```python
from build123d import *

# Parameters (mm, degrees)
SKETCH1_W                            = 159.7
SKETCH1_H                            = 109.7
SKETCH1_W_2                          = 143.7
SKETCH1_H_2                          = 102.7
BOSS_EXTRUDE1_DEPTH                  = 6
F_2_4_2_4_DIAMETER_HOLE1_D           = 2.4
CUT_EXTRUDE10_DEPTH                  = 2.2
LPATTERN1_COUNT                      = 2
LPATTERN1_PITCH                      = 72
MIRROR2_COPY_1_DEPTH                 = 2.2
M2X0_4_TAPPED_HOLE1_D                = 1.6
M2X0_4_TAPPED_HOLE1_DEPTH            = 3.5
M2X0_4_TAPPED_HOLE1_CSINK_D          = 2.05
M2X0_4_TAPPED_HOLE1_CSINK_ANGLE      = 90
M2X0_4_TAPPED_HOLE1_TIP              = 0.480688495
CUT_EXTRUDE3_DEPTH                   = 0.5
SKETCH11_W                           = 4.35
SKETCH11_H                           = 6
CUT_EXTRUDE4_DEPTH                   = 2.2
CUT_EXTRUDE11_DEPTH                  = 97.948362544
CUT_EXTRUDE11_DEPTH_BACK             = 97.948362544
F_2_4_2_4_DIAMETER_HOLE2_D           = 2.4
F_2_7_2_7_DIAMETER_HOLE1_D           = 2.7
F_2_7_2_7_DIAMETER_HOLE1_CSINK_D     = 2.75
F_2_7_2_7_DIAMETER_HOLE1_CSINK_ANGLE = 90
CUT_EXTRUDE6_DEPTH                   = 98.059492065
SKETCH19_R                           = 1.4
CUT_EXTRUDE7_DEPTH                   = 3.5
SKETCH32_R                           = 1.375
BOSS_EXTRUDE2_DEPTH                  = 1
CUT_EXTRUDE8_DEPTH                   = 98.126438213
SKETCH8_R                            = 8
CUT_EXTRUDE9_DEPTH                   = 98.126438213
FILLET1_R                            = 2
FILLET2_R                            = 8
FILLET3_R                            = 1
FILLET4_R                            = 2
FILLET5_R                            = 0.5
SKETCH31_W                           = 48
SKETCH31_H                           = 1.6
CUT_EXTRUDE12_DEPTH                  = 98.126438213
CHAMFER1_START                       = -1
CHAMFER1_DEPTH                       = 8
CHAMFER1_2_DEPTH                     = 6
FILLET6_R                            = 2


with BuildPart() as part:
    # Sketch1 → Boss-Extrude1 (new body)
    with BuildSketch(Plane(origin=(0, 0, 0), x_dir=(1, 0, 0), z_dir=(0, 1, 0))):
        Rectangle(SKETCH1_W, SKETCH1_H)
        Rectangle(SKETCH1_W_2, SKETCH1_H_2, mode=Mode.SUBTRACT)
    extrude(amount=BOSS_EXTRUDE1_DEPTH)

    # Ø2.4 (2.4) Diameter Hole1 (through all)
    with Locations(Plane(origin=(0, 6, 0), x_dir=(1, 0, 0), z_dir=(0, 1, 0))):
        with Locations((-77.5, 36), (77.5, 36), (-77.5, -36), (77.5, -36)):
            Hole(F_2_4_2_4_DIAMETER_HOLE1_D / 2)

    # Sketch29 → Cut-Extrude10 (cut)
    with BuildSketch(Plane(origin=(0, 6, 0), x_dir=(1, 0, 0), z_dir=(0, 1, 0))):
        with BuildLine():
            Line((-77.5, 38), (-79.85, 38))
            Line((-79.85, 38), (-79.85, 34))
            Line((-79.85, 34), (-77.5, 34))
            ThreePointArc((-77.5, 34), (-75.5, 36), (-77.5, 38))
        make_face()
    cut_extrude10 = extrude(amount=-CUT_EXTRUDE10_DEPTH, mode=Mode.SUBTRACT)

    # LPattern1: Cut-Extrude10 ×2
    with Locations(*[(0, 0, i * LPATTERN1_PITCH) for i in range(1, LPATTERN1_COUNT)]):
        add(cut_extrude10, mode=Mode.SUBTRACT)

    # Mirror2: Cut-Extrude10 across plane
    add(cut_extrude10.mirror(Plane(origin=(0, 0, 0), x_dir=(0, 0, 1), z_dir=(1, 0, 0))), mode=Mode.SUBTRACT)

    # Mirror2 copy 1 sketch → Mirror2 copy 1 (cut)
    with BuildSketch(Plane(origin=(0, 6, 72), x_dir=(-1, 0, 0), z_dir=(0, 1, 0))):
        with BuildLine():
            Line((-77.5, -38), (-79.85, -38))
            Line((-79.85, -38), (-79.85, -34))
            Line((-79.85, -34), (-77.5, -34))
            ThreePointArc((-77.5, -34), (-75.5, -36), (-77.5, -38))
        make_face()
    extrude(amount=-MIRROR2_COPY_1_DEPTH, mode=Mode.SUBTRACT)

    # M2x0.4 Tapped Hole1
    with Locations(Plane(origin=(0, 6, 0), x_dir=(1, 0, 0), z_dir=(0, 1, 0))):
        with Locations((-74, 40), (-74, -40), (74, 40), (74, -40)):
            CounterSinkHole(M2X0_4_TAPPED_HOLE1_D / 2, M2X0_4_TAPPED_HOLE1_CSINK_D / 2, depth=M2X0_4_TAPPED_HOLE1_DEPTH, counter_sink_angle=M2X0_4_TAPPED_HOLE1_CSINK_ANGLE)
            with Locations((0, 0, -(M2X0_4_TAPPED_HOLE1_DEPTH + M2X0_4_TAPPED_HOLE1_TIP / 2))):  # 118° drill point
                Cone(0, M2X0_4_TAPPED_HOLE1_D / 2, M2X0_4_TAPPED_HOLE1_TIP, mode=Mode.SUBTRACT)

    # Sketch9 → Cut-Extrude3 (cut)
    with BuildSketch(Plane(origin=(0, 6, 0), x_dir=(1, 0, 0), z_dir=(0, 1, 0))):
        with BuildLine():
            Line((-74.85, 4), (-74.85, -4))
            ThreePointArc((-74.85, -4), (-76.85, -6), (-78.85, -4))
            Line((-78.85, -4), (-78.85, 4))
            ThreePointArc((-78.85, 4), (-76.85, 6), (-74.85, 4))
        make_face()
    cut_extrude3 = extrude(amount=-CUT_EXTRUDE3_DEPTH, mode=Mode.SUBTRACT)

    # Mirror1: Cut-Extrude3 across plane
    add(cut_extrude3.mirror(Plane(origin=(0, 0, 0), x_dir=(0, 0, 1), z_dir=(1, 0, 0))), mode=Mode.SUBTRACT)

    # Sketch11 → Cut-Extrude4 (cut)
    with BuildSketch(Plane(origin=(0, 6, 0), x_dir=(1, 0, 0), z_dir=(0, 1, 0))):
        with Locations((-77.675, 39)):
            Rectangle(SKETCH11_W, SKETCH11_H)
    extrude(amount=-CUT_EXTRUDE4_DEPTH, mode=Mode.SUBTRACT)

    # Sketch30 → Cut-Extrude11 (cut, two sides: drawn at the far end of the back side and taken through both)
    with BuildSketch(Plane(origin=(0, 3.8, 0), x_dir=(1, 0, 0), z_dir=(0, 1, 0)).offset(-CUT_EXTRUDE11_DEPTH_BACK)):
        with BuildLine():
            Line((-75.5, 40), (-75.5, 42))
            Line((-75.5, 42), (-79.85, 42))
            Line((-79.85, 42), (-79.85, 38))
            Line((-79.85, 38), (-77.5, 38))
            ThreePointArc((-77.5, 38), (-76.085786438, 38.585786438), (-75.5, 40))
        make_face()
    extrude(amount=CUT_EXTRUDE11_DEPTH + CUT_EXTRUDE11_DEPTH_BACK, mode=Mode.SUBTRACT)

    # Ø2.4 (2.4) Diameter Hole2 (through all)
    with Locations(Plane(origin=(0, 6, 0), x_dir=(1, 0, 0), z_dir=(0, 1, 0))):
        with Locations((-77.5, -40), (77.5, 40), (77.5, -40)):
            Hole(F_2_4_2_4_DIAMETER_HOLE2_D / 2)

    # Ø2.7 (2.7) Diameter Hole1 (through all)
    with Locations(Plane(origin=(0, 6, 0), x_dir=(1, 0, 0), z_dir=(0, 1, 0))):
        with Locations((-77.5, 29), (-77.5, -29), (77.5, 29), (77.5, -29)):
            CounterSinkHole(F_2_7_2_7_DIAMETER_HOLE1_D / 2, F_2_7_2_7_DIAMETER_HOLE1_CSINK_D / 2, counter_sink_angle=F_2_7_2_7_DIAMETER_HOLE1_CSINK_ANGLE)

    # Sketch18 → Cut-Extrude6 (cut, through all)
    with BuildSketch(Plane(origin=(0, 6, 0), x_dir=(1, 0, 0), z_dir=(0, 1, 0))):
        with BuildLine():
            Line((-78.85, 24.85), (-79.85, 24.85))
            Line((-79.85, 24.85), (-79.85, 18.85))
            Line((-79.85, 18.85), (-78.85, 18.85))
            ThreePointArc((-78.85, 18.85), (-77.435786438, 19.435786438), (-76.85, 20.85))
            Line((-76.85, 20.85), (-76.85, 22.85))
            ThreePointArc((-76.85, 22.85), (-77.435786438, 24.264213562), (-78.85, 24.85))
        make_face()
    extrude(amount=-CUT_EXTRUDE6_DEPTH, mode=Mode.SUBTRACT)

    # Sketch19 → Cut-Extrude7 (cut)
    with BuildSketch(Plane(origin=(0, 6, 0), x_dir=(1, 0, 0), z_dir=(0, 1, 0))):
        with Locations(Location((77.35, 44.85, 0), (0, 0, 270))):
            Circle(SKETCH19_R)
        with Locations(Location((-77.35, -44.85, 0), (0, 0, 270))):
            Circle(SKETCH19_R)
    extrude(amount=-CUT_EXTRUDE7_DEPTH, mode=Mode.SUBTRACT)

    # Sketch32 → Boss-Extrude2 (add)
    with BuildSketch(Plane.XZ):
        with Locations(Location((-77.35, 44.85, 0), (0, 0, 90))):
            Circle(SKETCH32_R)
        with Locations(Location((77.35, -44.85, 0), (0, 0, 90))):
            Circle(SKETCH32_R)
    extrude(amount=BOSS_EXTRUDE2_DEPTH)

    # Sketch7 → Cut-Extrude8 (cut, through all)
    with BuildSketch(Plane(origin=(0, 6, 0), x_dir=(1, 0, 0), z_dir=(0, 1, 0))):
        with BuildLine():
            Line((-76.85, 48.85), (-79.85, 48.85))
            Line((-79.85, 48.85), (-79.85, 40.85))
            Line((-79.85, 40.85), (-76.85, 40.85))
            ThreePointArc((-76.85, 40.85), (-72.85, 44.85), (-76.85, 48.85))
        make_face()
    extrude(amount=-CUT_EXTRUDE8_DEPTH, mode=Mode.SUBTRACT)

    # Sketch8 → Cut-Extrude9 (cut, through all)
    with BuildSketch(Plane(origin=(0, 6, 0), x_dir=(1, 0, 0), z_dir=(0, 1, 0))):
        with Locations((-79.85, -54.85)):
            Circle(SKETCH8_R)
    extrude(amount=-CUT_EXTRUDE9_DEPTH, mode=Mode.SUBTRACT)

    # Fillet1
    fillet1_edges = [part.edges().sort_by_distance(p)[0] for p in [
        (71.85, 3, 51.35),
        (71.85, 3, -51.35),
        (-71.85, 3, -51.35),
        (-71.85, 3, 51.35),
    ]]
    fillet(fillet1_edges, radius=FILLET1_R)

    # Fillet2
    # the kernel refuses this fillet: 8 mm, written as the material it takes off along each edge
    with BuildSketch(Plane(origin=(79.85, -20, 54.85), x_dir=(-1, 0, 0), z_dir=(0, 1, 0)), Plane(origin=(79.85, -20, -54.85), x_dir=(0, 0, 1), z_dir=(0, 1, 0))) as fillet2_piece_1:
        with BuildLine():
            CenterArc((FILLET2_R, -FILLET2_R), FILLET2_R, 90, 90)
            Line((0, -FILLET2_R), (-FILLET2_R * 0.02, -FILLET2_R))
            Line((-FILLET2_R * 0.02, -FILLET2_R), (-FILLET2_R * 0.02, FILLET2_R * 0.02))
            Line((-FILLET2_R * 0.02, FILLET2_R * 0.02), (FILLET2_R, FILLET2_R * 0.02))
            Line((FILLET2_R, FILLET2_R * 0.02), (FILLET2_R, 0))
        make_face()
    extrude(amount=46, mode=Mode.SUBTRACT)
    with BuildSketch(Plane(origin=(-79.85, -19.364916731, -54.85), x_dir=(1, 0, 0), z_dir=(0, 1, 0))) as fillet2_piece_2:
        with BuildLine():
            CenterArc((7.745966692, -8), FILLET2_R, 90, 75.522487814)
            Line((0, -6), (-0.154919334, -5.96))
            ThreePointArc((-0.154919334, -5.96), (-0.16, -3), (-0.16, 0))
            Line((-0.16, 0), (0, 0.16))
            Line((0, 0.16), (7.745966692, 0.16))
            Line((7.745966692, 0.16), (7.745966692, 0))
        make_face()
    extrude(amount=44.729833462, mode=Mode.SUBTRACT)

    # Fillet3
    fillet3_edges = [part.edges().sort_by_distance(p)[0] for p in [
        (-79.85, 3, -48.85),
        (-71.85, 3, 54.85),
        (-79.85, 3, 46.85),
    ]]
    fillet(fillet3_edges, radius=FILLET3_R)

    # Fillet4
    fillet4_edges = [part.edges().sort_by_distance(p)[0] for p in [
        (-79.85, 1.9, -38),
    ]]
    fillet(fillet4_edges, radius=FILLET4_R)

    # Fillet5
    fillet5_edges = [part.edges().sort_by_distance(p)[0] for p in [
        (-79.85, 3, -18.85),
        (-79.85, 3, -24.85),
    ]]
    fillet(fillet5_edges, radius=FILLET5_R)

    # Sketch31 → Cut-Extrude12 (cut, through all)
    with BuildSketch(Plane(origin=(0, 6, 0), x_dir=(1, 0, 0), z_dir=(0, 1, 0))):
        with Locations((0, 52.15)):
            Rectangle(SKETCH31_W, SKETCH31_H)
    cut_extrude12 = extrude(amount=-CUT_EXTRUDE12_DEPTH, mode=Mode.SUBTRACT)

    # Mirror3: Cut-Extrude12 across plane
    add(cut_extrude12.mirror(Plane.XY), mode=Mode.SUBTRACT)

    # Chamfer1: read off the stored shape, not the designer's step
    # Chamfer1 outline → Chamfer1 (cut)
    with BuildSketch(Plane(origin=(0, 0, 0), x_dir=(1, 0, 0), z_dir=(0, 1, 0)).offset(CHAMFER1_START)):
        Polygon((25.6, 51.35), (24, 52.95), (24, 51.35), align=None)
        Polygon((-24, 52.95), (-25.6, 51.35), (-24, 51.35), align=None)
    extrude(amount=CHAMFER1_DEPTH, mode=Mode.SUBTRACT)

    # Chamfer1 2 outline → Chamfer1 2 (add)
    with BuildSketch(Plane(origin=(0, 0, 0), x_dir=(1, 0, 0), z_dir=(0, 1, 0))):
        Polygon((24, -52.95), (24, -51.35), (22.4, -52.95), align=None)
        Polygon((-24, -52.95), (-22.4, -52.95), (-24, -51.35), align=None)
    extrude(amount=CHAMFER1_2_DEPTH)

    # Fillet6
    fillet6_edges = [part.edges().sort_by_distance(p)[0] for p in [
        (-24, 3, -52.95),
        (24, 3, -52.95),
        (24, 3, 51.35),
        (-24, 3, 51.35),
        (-22.4, 3, 52.95),
        (22.4, 3, 52.95),
        (25.6, 3, -51.35),
        (-25.6, 3, -51.35),
    ]]
    fillet(fillet6_edges, radius=FILLET6_R)


solid = part.part
```
Design review of the part built by this model. Coordinates are the model's own, in mm. A direction names the side the tool comes from. Give positions to 0.01 mm unless a question says otherwise; leave off trailing zeros. Loops run counter-clockwise (first coordinate to the right, second up) from the corner with the lowest first, then second, coordinate; pieces in that order, holes last. Notation, with made-up numbers: (12, 19) -> (30, 19) arc R29 ccw to (30, 48) -> close; hole circle Ø6 at (78.5, 45). An arc over 180 degrees is marked (long way). One line per item, written item: value.
Q1. Draft analysis for pull direction X (two halves, no side actions). For faces 6 (the cylindrical face through (-76.327, 2.958, -53.645)), 7 (the flat face through (79, 3.8, -36)), 8 (the flat face through (77, 5.5, 0)), state which applies: pulls with the +X half, pulls with the -X half, needs draft (parallel to the pull), parting line crosses it, or undercut.
Numbers:
face 6: pulls with the -X half
face 7: needs draft
face 8: undercut
Q2. For pin 1 Ø1.8 at (x, y) = (78.5, 4.5) entering from -Z; pin 2 Ø1.7 at (x, y) = (-77.5, 3.5) entering from +Z; pin 3 Ø0.7 at (x, y) = (-78.5, 5) entering from +Z, all flat-tipped, find the tip position at first contact; note any pin that passes through.
Numbers:
pin 1: stops at z = -52.41
pin 2: stops at z = 47.52
pin 3: stops at z = 47.03
Q3. We need section A-A on x = 8. Give the boundary of the cut face in (y, z).
Numbers:
outline: (0, -54.85) -> (6, -54.85) -> (6, -52.95) -> (0, -52.95) -> close; (0, 52.95) -> (6, 52.95) -> (6, 54.85) -> (0, 54.85) -> close
Q4. Machinability: for faces 1 (the cylindrical face through (-74.14, 3.042, 49.247)), 2 (the flat face through (-79, 3.8, 36)), 3 (the flat face through (79, 3.8, 36)), 4 (the flat face through (-48, 3, 51.35)), 5 (the flat face through (79.85, 3, 1)), which of the approach directions +Z, -Z, +X, -X, +Y, -Y give a long, thin tool a straight path to every point of the face, cutting with its end or side? Answer none if there is none.
Numbers:
face 1: +Z, -X, +Y, -Y
face 2: -X, +Y
face 3: +X, +Y
face 4: +Y, -Y
face 5: +Z, -Z, +X, +Y, -Y
Q5. We need section B-B on z = 8. Give the boundary of the cut face in (x, y), and give its area (3 significant figures).
Numbers:
outline: (-79.85, 0) -> (-71.85, 0) -> (-71.85, 6) -> (-79.85, 6) -> close; (71.85, 0) -> (79.85, 0) -> (79.85, 6) -> (71.85, 6) -> close
area: 96.0 mm^2
Q6. For L1, parallel to X at y = 1.5, z = -36; L2, parallel to X at y = 4.8, z = 40; L3, parallel to X at y = 4.4, z = 29, list the stretches that pass through material, from the lowest coordinate up.
Numbers:
L1: x = -79.85 to -78.7, -76.3 to -71.85, 71.85 to 76.3, 78.7 to 79.85
L2: x = -79.85 to -78.7, -76.3 to -74.8, -73.2 to -71.85, 71.85 to 73.2, 74.8 to 76.3, 78.7 to 79.85
L3: x = -79.85 to -78.85, -76.15 to -71.85, 71.85 to 76.15, 78.85 to 79.85
